from build123d import *


# Not quite as in the source:
# - a feature of the source that left no trace in its solid (it failed there, or was rolled back) is left out


with BuildPart() as f1:
    # F0 (on Front) → F1 (revolve)
    with BuildSketch(Plane.XZ):
        with BuildLine():
            Line((0, 43.3218007376), (0, 0))
            Line((0, 0), (48, 0))
            Line((48, 0), (48, 69))
            Line((48, 69), (33, 69))
            Line((33, 69), (33, 60))
            Line((33, 60), (30.3564090981, 60))
            ThreePointArc((30.3564090981, 60), (28.9421955357, 59.4142135624), (28.3564090981, 58))
            Line((28.3564090981, 58), (28.3564090981, 50))
            Line((28.3564090981, 50), (1.6527036447, 45.2914162437))
            ThreePointArc((1.6527036447, 45.2914162437), (0.4679111138, 44.607375957), (0, 43.3218007376))
        make_face()
    revolve(axis=Axis((24, 0, 0), (-1, 0, 0)))


solid = f1.part
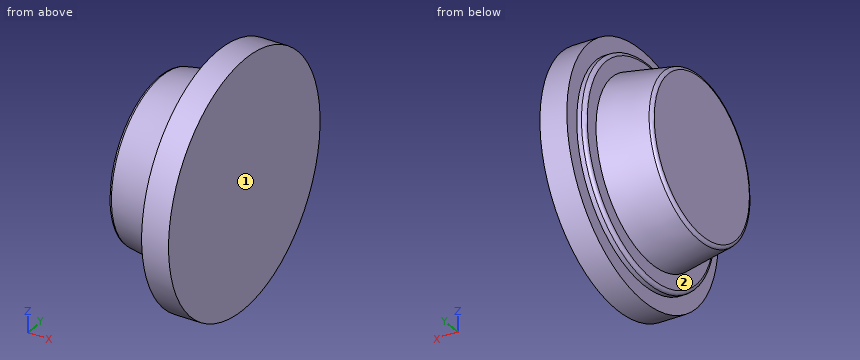
For this review, take the finished solid that the model builds, in its own axes (mm). Face numbers are marked on the shaded views. A direction names the side the tool comes from. Coordinates: 2 decimals unless noted, no trailing zeros. Loops run counter-clockwise (first coordinate to the right, second up) from the corner with the lowest first, then second, coordinate; pieces in that order, holes last. Notation, with made-up numbers: (79, 26.5) - (86, 26.5) arc R24 cw to (86, 45.5) - close; hole circle Ø6 at (41.5, 83.25). An arc over 180 degrees is marked (long way). Use a Markdown table: item, result. Add a question column.
Item 1: We need section A-A (z = 0). Give the boundary of the cut face in (x, y).
Item 2: Insertion check: pin 1 Ø1.5 at (x, z) = (20.5, -41.5) entering from -Y; pin 2 Ø5 at (x, y) = (16.5, 15) entering from +Z; pin 3 Ø1 at (x, z) = (24, 34) entering from -Y. Each pin has a flat end and moves straight along its axis. Give the tip position at first contact, or say it passes through.
Item 3: Tool access review of the marked faces 1 and 2: name each direction out of +Z, -Z, +X, -X, +Y, -Y from which nothing blocks a thin tool from reaching the whole face with its end or side.
Item 4: For line 1 (X direction, y = -47.5, z = 40); line 2 (X direction, y = -54, z = 20); line 3 (Z direction, x = 32, y = 3.5), list the stretches that pass through material, from the lowest coordinate up.
Item 5: We need section D-D (x = 12.5). Give the boundary of the cut face in (y, z).
Item 6: We need section C-C (x = 35). Give the boundary of the cut face in (y, z).
Results list:
| question | item | result |
|---|---|---|
| 1 | outline | (0, -43.32) arc R2 ccw to (1.65, -45.29) - (28.36, -50) - (28.36, -58) arc R2 ccw to (30.36, -60) - (33, -60) - (33, -69) - (48, -69) - (48, 69) - (33, 69) - (33, 60) - (30.36, 60) arc R2 ccw to (28.36, 58) - (28.36, 50) - (1.65, 45.29) arc R2 ccw to (0, 43.32) - close |
| 2 | pin 1 | stops at y = -26.54 |
| 2 | pin 2 | stops at z = 46.39 |
| 2 | pin 3 | stops at y = -36.09 |
| 3 | face 1 | +Z, -Z, +X, +Y, -Y |
| 3 | face 2 | -X |
| 4 | line 1 | x = 33 to 48 |
| 4 | line 2 | x = 28.36 to 48 |
| 4 | line 3 | z = -59.9 to 59.9 |
| 5 | outline | circle Ø94.41 at (0, 0) |
| 6 | outline | circle Ø138 at (0, 0) |
